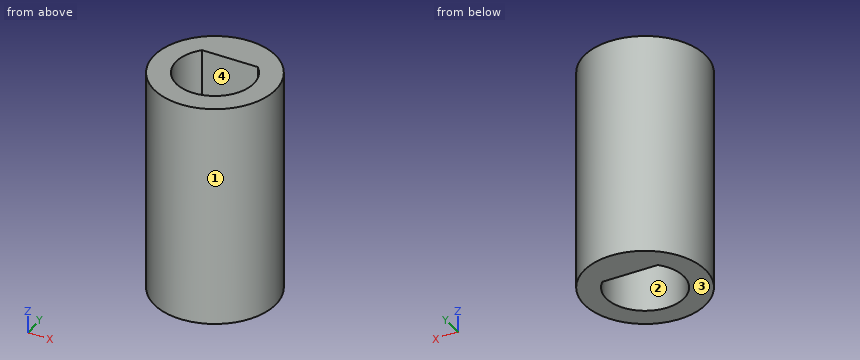
Autodesk Inventor part; units mm, degrees
sketch "Sketch1" plane through (0, 0, 0) normal (0, 0, 1) x (1, 0, 0)
  circle A0 centre (0, 0) radius 2.5
  line L0 (-1.118, 1) -> (1.118, 1)
  arc A1 (-1.118, 1) -> (1.118, 1) centre (0, 0) ccw
  line L1 (-1.1619, 1.1) -> (1.1619, 1.1)
  arc A2 (-1.1619, 1.1) -> (1.1619, 1.1) centre (0, 0) ccw
  dimension "d1" = 3.2
  dimension "d0" = 5
  dimension "d4" = 0.5
extrude "Extrusion2" add sketch "Sketch1" along normal mid plane 9.2 contours A0
properties part number "conector_motor_001" material "ABS Plastic"
Work out the finished part from the listing and answer in its coordinate system (mm). Face numbers are marked on the shaded views. Give positions to 0.01 mm unless a question says otherwise; leave off trailing zeros. Loops run counter-clockwise (first coordinate to the right, second up) from the corner with the lowest first, then second, coordinate; pieces in that order, holes last. Notation, with made-up numbers: (-19, 69.25) - (-5, 69.25) arc R34 cw to (-5, 99.25) - close; hole circle Ø6 at (50, 69). An arc over 180 degrees is marked (long way). Answer in a Markdown table with one row per item. Add a question column.
Q1. The part is cut by section D-D (y = -2). Determine the outline of the cut face in (x, z).
Q2. Determine the mould class of the marked faces 1, 2, 3 and 4 for opening direction Y: released by +Y, released by -Y, zero draft, split by the parting line, or undercut.
Q3. The part is cut by section A-A (y = 0). Determine the outline of the cut face in (x, z), and give its area (3 significant figures).
Q4. The part is cut by section C-C (z = 3.25). Determine the outline of the cut face in (x, y).
Q5. The part is cut by section B-B (x = 0). Determine the outline of the cut face in (y, z).
Q6. Consider line 1 along Y through (x, z) = (0.1, 3); line 2 along X through (y, z) = (0.55, -3); line 3 along X through (y, z) = (0.95, -3). Determine where each line is inside the solid, lowest interval first.
Q7. Each of these flat-tipped pins is pushed along its axis until it touches: P1, Ø2, axis at x = 0.5, y = -1, coming from the +Z side; P2, Ø1.9, axis at x = 0, y = 0, coming from the +Z side; P3, Ø3, axis at x = -2, z = 1.5, coming from the +Y side. Where does it stop, or does it pass through?
Solution:
| question | item | result |
|---|---|---|
| 1 | outline | (-1.5, -4.6) - (1.5, -4.6) - (1.5, 4.6) - (-1.5, 4.6) - close |
| 2 | face 1 | split by the parting line |
| 2 | face 2 | undercut |
| 2 | face 3 | zero draft |
| 2 | face 4 | undercut |
| 3 | outline | (-2.5, -4.6) - (-1.6, -4.6) - (-1.6, 4.6) - (-2.5, 4.6) - close; (1.6, -4.6) - (2.5, -4.6) - (2.5, 4.6) - (1.6, 4.6) - close |
| 3 | area | 16.6 mm² |
| 4 | outline | circle Ø5 at (0, 0); hole (-1.16, 1.1) arc R1.6 ccw (long way) to (1.16, 1.1) - close |
| 5 | outline | (-2.5, -4.6) - (-1.6, -4.6) - (-1.6, 4.6) - (-2.5, 4.6) - close; (1.1, -4.6) - (2.5, -4.6) - (2.5, 4.6) - (1.1, 4.6) - close |
| 6 | line 1 | y = -2.5 to -1.6, 1.1 to 2.5 |
| 6 | line 2 | x = -2.44 to -1.5, 1.5 to 2.44 |
| 6 | line 3 | x = -2.31 to -1.29, 1.29 to 2.31 |
| 7 | P1 | stops at z = 4.6 |
| 7 | P2 | passes through |
| 7 | P3 | stops at y = 2.45 |
